```python
from build123d import *

# Parameters (mm, degrees)
F0_R     = 75
F0_R_2   = 9
F0_R_3   = 20
F1_DEPTH = 15
F2_R     = 35
F2_R_2   = 20
F3_DEPTH = 68
F4_R     = 75
F4_R_2   = 9
F4_R_3   = 20
F5_DEPTH = 15


with BuildPart() as f1:
    # F0 (on Top) → F1 (new body)
    with BuildSketch(Plane.XY):
        Circle(F0_R)
        with Locations((0, -55)):
            Circle(F0_R_2, mode=Mode.SUBTRACT)
        with Locations((-55, 0)):
            Circle(F0_R_2, mode=Mode.SUBTRACT)
        Circle(F0_R_3, mode=Mode.SUBTRACT)
        with Locations((55, 0)):
            Circle(F0_R_2, mode=Mode.SUBTRACT)
        with Locations((0, 55)):
            Circle(F0_R_2, mode=Mode.SUBTRACT)
    extrude(amount=F1_DEPTH)

    # F2 (on face) → F3 (join)
    with BuildSketch(Plane.XY.offset(15)):
        Circle(F2_R)
        Circle(F2_R_2, mode=Mode.SUBTRACT)
    extrude(amount=F3_DEPTH)

    # F4 (on face) → F5 (join)
    with BuildSketch(Plane.XY.offset(83)):
        Circle(F4_R)
        with Locations((0, -55)):
            Circle(F4_R_2, mode=Mode.SUBTRACT)
        with Locations((-55, 0)):
            Circle(F4_R_2, mode=Mode.SUBTRACT)
        Circle(F4_R_3, mode=Mode.SUBTRACT)
        with Locations((55, 0)):
            Circle(F4_R_2, mode=Mode.SUBTRACT)
        with Locations((0, 55)):
            Circle(F4_R_2, mode=Mode.SUBTRACT)
    extrude(amount=F5_DEPTH)


solid = f1.part
```
Verification items for the finished model (mm, model axes). A direction names the side the tool comes from. Coordinates: 2 decimals unless noted, no trailing zeros. Write each loop counter-clockwise with the first axis right and the second up, starting at its lowest first coordinate (ties: lowest second). Pieces come first, ordered by that corner, then holes. Notation, with made-up numbers: (-37, 2) - (2, 2) arc R14 cw to (2, 19) - close; hole circle Ø11 at (19, 18). An arc over 180 degrees is marked (long way). Write item = value, one per line.
Q1. Cross-section at C-C (y = -55). Enter the section's corners in (x, z), plus the area to 3 significant figures.
Answer:
outline = (-50.99, 0) - (-9, 0) - (-9, 15) - (-50.99, 15) - close; (-50.99, 83) - (-9, 83) - (-9, 98) - (-50.99, 98) - close; (9, 0) - (50.99, 0) - (50.99, 15) - (9, 15) - close; (9, 83) - (50.99, 83) - (50.99, 98) - (9, 98) - close
area = 2,520 mm²
Q2. Mould release check, pull along X, two halves, no side actions. Record for faces 3 (the face through (53.828, 8.923, 7.395)), 4 (the face through (32, -16, 15)), 5 (the face through (-9.764, 74.362, 7.395)), 6 (the face through (4.84, 62.59, 7.4)): released by +X, released by -X, zero draft, split by the parting line, or undercut.
Answer:
face_3 = undercut
face_4 = zero draft
face_5 = split by the parting line
face_6 = undercut
Q3. Go/stop test with flat-tipped pins: pin 1 Ø16 at (x, y) = (-55, 0) entering from +Z (3 decimals); pin 2 Ø3 at (y, z) = (24.5, 49.5) entering from -X; pin 3 Ø10 at (x, z) = (0, 43) entering from +Y; pin 4 Ø4 at (x, z) = (-24, 78) entering from -Y. Record where each tip stops, or that it passes through.
Answer:
pin_1 = through
pin_2 = -26.38
pin_3 = 35
pin_4 = -27.22
Q4. Material ranges on L1, parallel to Y at x = 0, z = 91; L2, parallel to Z at x = -64, y = -38.5; L3, parallel to Y at x = 6.5, z = 10, recorded low to high. Write a range as from..to.
Answer:
L1 = -75..-64, -46..-20, 20..46, 64..75
L2 = 0..15, 83..98
L3 = -74.72..-61.22, -48.78..-18.91, 18.91..48.78, 61.22..74.72
Q5. Cross-section at D-D (x = -17). Enter the section's corners in (y, z).
Answer:
outline = (-73.05, 0) - (-10.54, 0) - (-10.54, 98) - (-73.05, 98) - (-73.05, 83) - (-30.59, 83) - (-30.59, 15) - (-73.05, 15) - close; (10.54, 0) - (73.05, 0) - (73.05, 15) - (30.59, 15) - (30.59, 83) - (73.05, 83) - (73.05, 98) - (10.54, 98) - close
Q6. Cross-section at A-A (x = 0). Give the number of separate pieces and of enclosed holes in the cut face, plus the area to 3 significant figures.
Answer:
separate_pieces = 6
enclosed_holes = 0
area = 4,260 mm²
Q7. Access from +Z, -Z, +X, -X, +Y, -Y to the whole of each face (thin tool, end or side, straight path). Record for faces 1 (the face through (53.828, 8.923, 90.395)), 2 (the face through (32, -16, 83)).
Answer:
face_1 = +Z, -Z
face_2 = none
